Autodesk Inventor part; units mm, degrees
ref_plane "YZ Plane" through (0, 0, 0) normal (1, 0, 0) x (0, 1, 0)
ref_plane "XZ Plane" through (0, 0, 0) normal (0, 1, 0) x (-1, 0, 0)
ref_plane "XY Plane" through (0, 0, 0) normal (0, 0, 1) x (1, 0, 0)
sketch "Sketch1" plane through (0, 0, 0) normal (0, 0, 1) x (1, 0, 0)
  circle A0 centre (0, 0) radius 6.5
  ellipse E0 centre (17.3675, 0) end of major axis (34.735, 0) minor radius 5.08
  line L0 (0, 30.8967) -> (0, 25.9123)
  ellipse E1 centre (-17.3675, 0) end of major axis (-34.735, 0) minor radius 5.08
  circle A1 centre (0, 0) radius 1
  circle A2 centre (0, 0) radius 1.6425
  circle A3 centre (0, 0) radius 2.3228
  dimension "d1" = 17.3675
  dimension "d2" = 5.08
  dimension "d0" = 13
  dimension "d7" = 2
extrude "Extrusion1" add sketch "Sketch1" along normal mid plane 6.93 contours A0 E0 A3 | E0 A3 E1 A0 | A0 E1 A3 E0 | E1 A3 A0 | A3 E0 A2 | E0 A2 E1 A3 | A3 E1 A2 E0 | E1 A2 A3 | A2 E0 A1 | E0 A1 E1 A2 | A2 E1 A1 E0 | E1 A1 A2 | A1 E0 | E0 E1 A1 | A1 E1 E0 | E1 A1
extrude "Extrusion2" add sketch "Sketch1" along normal blind 2 contours A0 E0 A3 | A0 E0 | E1 A3 A0 | A0 E1 | A3 E0 A2 | E1 A2 A3 | A2 E0 A1 | E1 A1 A2 | A1 E0 | E1 A1
extrude "Extrusion3" cut sketch "Sketch1" along normal through all both and the other way through all contours A1 E0 | E0 E1 A1 | A1 E1 E0 | E1 A1
extrude "Extrusion4" cut sketch "Sketch1" along normal blind 1 contours A2 E0 A1 | E0 A1 E1 A2 | A2 E1 A1 E0 | E1 A1 A2
extrude "Extrusion5" cut sketch "Sketch1" along normal blind 2 contours A3 E0 A2 | E0 A2 E1 A3 | A3 E1 A2 E0 | E1 A2 A3
sketch "Sketch2" plane through (0, 0, 2) normal (0, 0, 1) x (1, 0, 0)
  point P0 (0, 0)
properties part number "Baling2"
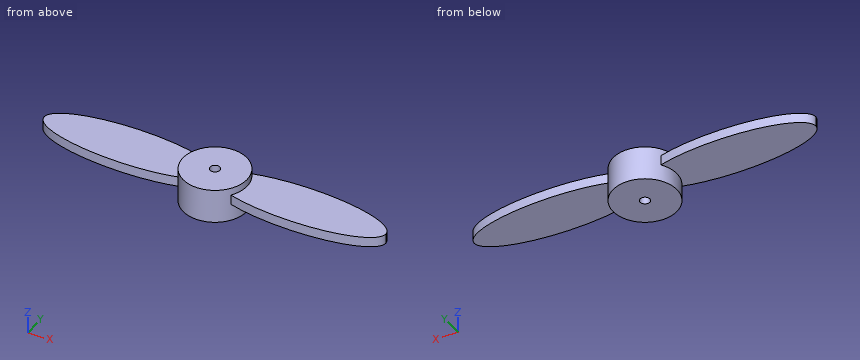
Can you work these out from the model? Positions are in its coordinate system, mm. Give positions to 0.01 mm unless a question says otherwise; leave off trailing zeros. Loops run counter-clockwise (first coordinate to the right, second up) from the corner with the lowest first, then second, coordinate; pieces in that order, holes last. Notation, with made-up numbers: (-11, -25.5) - (-1, -25.5) arc R34 cw to (-1, 4.5) - close; hole circle Ø7 at (-13, 39). An arc over 180 degrees is marked (long way). One line per item, written item: value.
(1) I need wall thicknesses on line 1 along Y through (x, z) = (0, 1.3); line 2 along X through (y, z) = (0, 2.3); line 3 along X through (y, z) = (-1.5, 1.75). Which ranges of each line are inside material? Lowest first, please.
Verdict:
line 1: -6.5 to -2.32, -1.64 to -1, 1 to 1.64, 2.32 to 6.5
line 2: -6.5 to -1, 1 to 6.5
line 3: -33.96 to -1.77, -0.67 to 0.67, 1.77 to 33.96
(2) I'm going to push flat-ended pins straight in: pin 1 (5 mm diameter, centred on x = 0, y = -0.5, fed in from +Z) (3 decimals); pin 2 (5 mm diameter, centred on x = -17, y = 0, fed in from -Z); pin 3 (3 mm diameter, centred on x = 10, z = 2.5, fed in from +Y); pin 4 (4 mm diameter, centred on x = 18.5, z = 0, fed in from +Y). Where does each tip first touch, or does it pass through?
Verdict:
pin 1: z = 3.465
pin 2: z = 0
pin 3: y = 4.77
pin 4: y = 5.08
(3) If we section it at A-A, the plane x = 0: List the corners of the cut face in (y, z) for me (1 decimal), plus the area to 3 significant figures.
Verdict:
outline: (-6.5, -3.5) - (-1, -3.5) - (-1, 0) - (-2.3, 0) - (-2.3, 2) - (-1.6, 2) - (-1.6, 1) - (-1, 1) - (-1, 3.5) - (-6.5, 3.5) - close; (1, -3.5) - (6.5, -3.5) - (6.5, 3.5) - (1, 3.5) - (1, 1) - (1.6, 1) - (1.6, 2) - (2.3, 2) - (2.3, 0) - (1, 0) - close
area: 72.2 mm^2
